Read the model definition and answer for the solid it produces. Units are mm, in the model's axes. Face numbers are marked on the shaded views. A direction names the side the tool comes from. Round coordinates to 2 decimals unless told otherwise and drop trailing zeros. Loops run counter-clockwise (first coordinate to the right, second up) from the corner with the lowest first, then second, coordinate; pieces in that order, holes last. Notation, with made-up numbers: (61, -18) - (105, -18) arc R22 ccw to (105, 15) - close; hole circle Ø11 at (29.5, -11). An arc over 180 degrees is marked (long way). Answer as CSV lines item,"result".
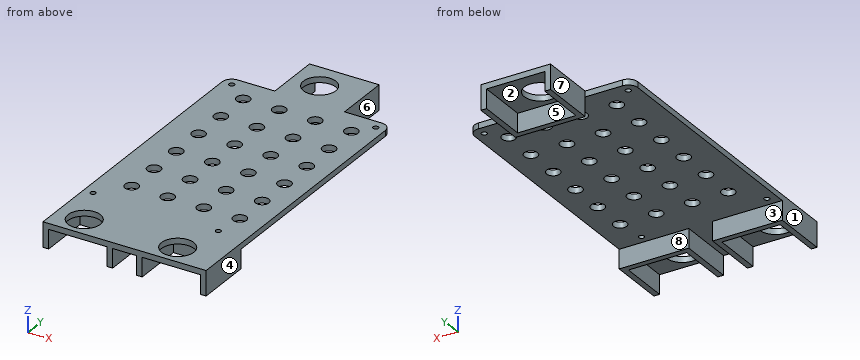
Autodesk Inventor part; units mm, degrees
ref_plane "Arbeitsebene2" through (-15.25, 66.75, 0) normal (0, 0, 1) x (1, 0, 0)
ref_plane "YZ Plane" through (0, 0, 0) normal (1, 0, 0) x (0, 1, 0)
ref_plane "XZ Plane" through (0, 0, 0) normal (0, 1, 0) x (-1, 0, 0)
ref_plane "Arbeitsebene1" through (0, 0, 0) normal (0, 0, 1) x (1, 0, 0)
sketch "Skizze1" plane through (0, 0, 0) normal (0, 0, 1) x (1, 0, 0)
  arc A0 (-36.75, 55.75) -> (-34.75, 57.75) centre (-36.75, 57.75) ccw
  line L0 (-34.75, 57.75) -> (-34.75, 60.25)
  arc A1 (-32.75, 62.25) -> (-34.75, 60.25) centre (-32.75, 60.25) ccw
  line L1 (-32.75, 62.25) -> (32.25, 62.25)
  arc A2 (34.25, 60.25) -> (32.25, 62.25) centre (32.25, 60.25) ccw
  line L2 (34.25, 60.25) -> (34.25, 57.25)
  arc A3 (34.25, 57.25) -> (36.25, 55.25) centre (36.25, 57.25) ccw
  line L3 (36.25, 55.25) -> (39.25, 55.25)
  arc A4 (41.25, 53.25) -> (39.25, 55.25) centre (39.25, 53.25) ccw
  line L4 (41.25, 53.25) -> (41.25, -58.75)
  arc A5 (37.75, -62.25) -> (41.25, -58.75) centre (37.75, -58.75) ccw
  line L5 (37.75, -62.25) -> (33.25, -62.25)
  arc A6 (31.25, -60.25) -> (33.25, -62.25) centre (33.25, -60.25) ccw
  line L6 (31.25, -60.25) -> (31.25, -57.25)
  arc A7 (31.25, -57.25) -> (29.25, -55.25) centre (29.25, -57.25) ccw
  line L7 (29.25, -55.25) -> (26.25, -55.25)
  arc A8 (26.25, -55.25) -> (24.25, -57.25) centre (26.25, -57.25) ccw
  line L8 (24.25, -57.25) -> (24.25, -60.25)
  arc A9 (22.25, -62.25) -> (24.25, -60.25) centre (22.25, -60.25) ccw
  line L9 (22.25, -62.25) -> (-30.5541, -62.25)
  arc A10 (-32.5541, -60.25) -> (-30.5541, -62.25) centre (-30.5541, -60.25) ccw
  line L10 (-32.5541, -60.25) -> (-32.5541, -56.8048)
  arc A11 (-32.5541, -56.8048) -> (-34.5541, -54.8048) centre (-34.5541, -56.8048) ccw
  line L11 (-34.5541, -54.8048) -> (-39.25, -54.8048)
  arc A12 (-41.25, -52.8048) -> (-39.25, -54.8048) centre (-39.25, -52.8048) ccw
  line L12 (-41.25, -52.8048) -> (-41.25, 53.75)
  arc A13 (-39.25, 55.75) -> (-41.25, 53.75) centre (-39.25, 53.75) ccw
  line L13 (-39.25, 55.75) -> (-36.75, 55.75)
  line L14 (42.75, -58.75) -> (42.75, 58.75)
  arc A14 (42.75, 58.75) -> (37.75, 63.75) centre (37.75, 58.75) ccw
  line L15 (37.75, 63.75) -> (-37.75, 63.75)
  arc A15 (-37.75, 63.75) -> (-42.75, 58.75) centre (-37.75, 58.75) ccw
  line L16 (-42.75, 58.75) -> (-42.75, -58.75)
  arc A16 (-42.75, -58.75) -> (-37.75, -63.75) centre (-37.75, -58.75) ccw
  line L17 (-37.75, -63.75) -> (37.75, -63.75)
  arc A17 (37.75, -63.75) -> (42.75, -58.75) centre (37.75, -58.75) ccw
  circle A18 centre (-37.75, 58.75) radius 1.4
  circle A19 centre (-37.75, -58.75) radius 1.4
  circle A20 centre (37.75, 58.75) radius 1.4
  circle A21 centre (28.25, -59.25) radius 1.4
  point P0 (0, 0)
extrude "Extrusion1" add sketch "Skizze1" along normal blind 3 contours A0 L0 A1 L1 A2 L2 A3 L3 A4 L4 A5 L5 A6 L6 A7 L7 A8 L8 A9 L9 A10 L10 A11 L11 A12 L12 A13 L13 | A17 L17 A16 L16 A15 L15 A14 L14
sketch "Skizze2" plane through (0, 0, 3) normal (0, 0, 1) x (1, 0, 0)
  circle A0 centre (-26.4114, 50.1197) radius 3.8655 construction
  circle A1 centre (-26.4114, 50.1197) radius 3.5
  point P0 (0, 0)
  dimension "d2" = 7
extrude "Extrusion2" cut sketch "Skizze2" against normal through all
pattern_linear "Rechteckige Anordnung1" count 6 spacing 18.9 along (0, -1, 0) count 4 spacing 18.9 along (1, 0, 0) of "Extrusion2"
sketch "Skizze3" plane through (0, 0, 3) normal (0, 0, 1) x (1, 0, 0)
  circle A0 centre (-28.25, -81.65) radius 8.5
  line L0 (-9.25, -66.75) -> (-39.75, -66.75)
  line L1 (-39.75, -66.75) -> (-39.75, -93.15)
  line L2 (-39.75, -93.15) -> (-9.25, -93.15)
  line L3 (-9.25, -93.15) -> (-9.25, -66.75)
  circle A1 centre (-3.75, 78.25) radius 8.5
  line L4 (15.25, 93.15) -> (-15.25, 93.15)
  line L5 (-15.25, 93.15) -> (-15.25, 66.75)
  line L6 (-15.25, 66.75) -> (15.25, 66.75)
  line L7 (15.25, 66.75) -> (15.25, 93.15)
  circle A2 centre (20.75, -81.65) radius 8.5
  line L8 (39.75, -66.75) -> (9.25, -66.75)
  line L9 (9.25, -66.75) -> (9.25, -93.15)
  line L10 (9.25, -93.15) -> (39.75, -93.15)
  line L11 (39.75, -93.15) -> (39.75, -66.75)
  line L12 (-42.75, 58.75) -> (-42.75, -58.75)
  line L13 (-42.75, -66.75) -> (-42.75, -58.75)
  line L14 (-42.75, -58.75) -> (-41.9493, -58.75)
  line L15 (-9.25, -93.15) -> (9.25, -93.15)
  arc A3 (37.75, -63.75) -> (42.75, -58.75) centre (37.75, -58.75) ccw
  line L16 (42.75, -66.75) -> (42.75, -58.75)
  line L17 (37.75, 63.75) -> (-37.75, 63.75)
  line L18 (-15.25, 93.15) -> (15.25, 93.15)
  line L19 (15.25, 93.15) -> (15.25, 63.75)
  line L20 (15.25, 63.75) -> (-15.25, 63.75)
  line L21 (-15.25, 63.75) -> (-15.25, 93.15)
  arc A4 (-42.75, -58.75) -> (-37.75, -63.75) centre (-37.75, -58.75) ccw
  circle A5 centre (30.2886, -44.3803) radius 3.5
  circle A6 centre (30.2886, -25.4803) radius 3.5
  circle A7 centre (30.2886, -6.5803) radius 3.5
  circle A8 centre (30.2886, 12.3197) radius 3.5
  circle A9 centre (30.2886, 31.2197) radius 3.5
  circle A10 centre (30.2886, 50.1197) radius 3.5
  circle A11 centre (11.3886, -44.3803) radius 3.5
  circle A12 centre (11.3886, -25.4803) radius 3.5
  circle A13 centre (11.3886, -6.5803) radius 3.5
  circle A14 centre (11.3886, 12.3197) radius 3.5
  circle A15 centre (11.3886, 31.2197) radius 3.5
  circle A16 centre (11.3886, 50.1197) radius 3.5
  circle A17 centre (-7.5114, -44.3803) radius 3.5
  circle A18 centre (-7.5114, -25.4803) radius 3.5
  circle A19 centre (-7.5114, -6.5803) radius 3.5
  circle A20 centre (-7.5114, 12.3197) radius 3.5
  circle A21 centre (-7.5114, 31.2197) radius 3.5
  circle A22 centre (-7.5114, 50.1197) radius 3.5
  circle A23 centre (-26.4114, -44.3803) radius 3.5
  circle A24 centre (-26.4114, -25.4803) radius 3.5
  circle A25 centre (-26.4114, -6.5803) radius 3.5
  circle A26 centre (-26.4114, 12.3197) radius 3.5
  circle A27 centre (-26.4114, 31.2197) radius 3.5
  circle A28 centre (-26.4114, 50.1197) radius 3.5
  arc A29 (42.75, 58.75) -> (37.75, 63.75) centre (37.75, 58.75) ccw
  line L22 (37.75, 63.75) -> (-37.75, 63.75)
  arc A30 (-37.75, 63.75) -> (-42.75, 58.75) centre (-37.75, 58.75) ccw
  line L23 (-42.75, 58.75) -> (-42.75, -58.75)
  arc A31 (-42.75, -58.75) -> (-37.75, -63.75) centre (-37.75, -58.75) ccw
  line L24 (-37.75, -63.75) -> (37.75, -63.75)
  arc A32 (37.75, -63.75) -> (42.75, -58.75) centre (37.75, -58.75) ccw
  line L25 (42.75, -58.75) -> (42.75, 58.75)
  circle A33 centre (28.25, -59.25) radius 1.4
  circle A34 centre (37.75, 58.75) radius 1.4
  circle A35 centre (-37.75, -58.75) radius 1.4
  circle A36 centre (-37.75, 58.75) radius 1.4
  line L26 (15.25, 93.15) -> (18.25, 93.15)
  line L27 (18.25, 93.15) -> (18.25, 63.75)
  line L28 (18.25, 63.75) -> (15.25, 63.75)
  line L29 (15.25, 63.75) -> (15.25, 93.15)
  line L30 (-15.25, 93.15) -> (-18.25, 93.15)
  line L31 (-18.25, 93.15) -> (-18.25, 63.75)
  line L32 (-18.25, 63.75) -> (-15.25, 63.75)
  line L33 (-15.25, 63.75) -> (-15.25, 93.15)
  line L34 (-39.75, -93.15) -> (-42.75, -93.15)
  line L35 (-42.75, -93.15) -> (-42.75, -58.75)
  line L36 (-42.75, -58.75) -> (-39.75, -58.75)
  line L37 (-39.75, -58.75) -> (-39.75, -93.15)
  line L38 (39.75, -93.15) -> (42.75, -93.15)
  line L39 (42.75, -93.15) -> (42.75, -58.75)
  line L40 (42.75, -58.75) -> (39.75, -58.75)
  line L41 (39.75, -58.75) -> (39.75, -93.15)
  point P0 (0, 0)
  point P1 (15.25, 66.75)
  point P2 (-15.25, 63.75)
  point P3 (41.5171, -62.0377)
  point P4 (42.75, -58.75)
  point P5 (42.75, -58.75)
  point P6 (-41.5171, -62.0377)
  point P7 (42.75, -58.75)
  point P8 (41.5171, -62.0377)
  point P9 (42.75, -58.75)
  point P10 (-37.75, 63.75)
  dimension "d17" = 3
  dimension "d18" = 3
ref_plane "Arbeitsebene2" through (-15.25, 66.75, 0) normal (0, 0, 1) x (1, 0, 0)
extrude "Extrusion3" add sketch "Skizze3" against normal up to surface (3 mm away)
sketch "Skizze4" plane through (0, 0, 0) normal (0, 0, -1) x (-1, 0, 0)
  circle A0 centre (19.25, -88.65) radius 0.65
  line L0 (9.25, -93.15) -> (9.25, -66.75)
  line L1 (9.25, -66.75) -> (39.75, -66.75)
  line L2 (-9.25, -66.75) -> (-9.25, -93.15)
  line L3 (-39.75, -66.75) -> (-9.25, -66.75)
  line L4 (15.25, 66.75) -> (-15.25, 66.75)
  line L5 (-37.75, 63.75) -> (37.75, 63.75)
  line L6 (-15.25, 66.75) -> (15.25, 66.75)
  line L7 (15.25, 66.75) -> (15.25, 63.75)
  line L8 (15.25, 63.75) -> (-15.25, 63.75)
  line L9 (-15.25, 63.75) -> (-15.25, 66.75)
  line L10 (9.25, -93.15) -> (6.25, -93.15)
  line L11 (6.25, -93.15) -> (6.25, -63.7252)
  line L12 (6.25, -63.7252) -> (9.25, -63.7252)
  line L13 (9.25, -63.7252) -> (9.25, -93.15)
  line L14 (-9.25, -93.15) -> (-6.25, -93.15)
  line L15 (-6.25, -93.15) -> (-6.25, -63.7252)
  line L16 (-6.25, -63.7252) -> (-9.25, -63.7252)
  line L17 (-9.25, -63.7252) -> (-9.25, -93.15)
  line L18 (42.75, 58.75) -> (42.75, -93.15)
  line L19 (-42.75, 58.75) -> (-42.75, -93.15)
  line L20 (-9.25, -66.75) -> (-39.75, -66.75)
  line L21 (-39.75, -66.75) -> (-39.75, -63.7252)
  line L22 (-39.75, -63.7252) -> (-9.25, -63.7252)
  line L23 (-9.25, -63.7252) -> (-9.25, -66.75)
  line L24 (42.75, 58.75) -> (42.75, -93.15)
  line L25 (9.25, -66.75) -> (42.75, -66.75)
  line L26 (42.75, -66.75) -> (42.75, -63.7252)
  line L27 (42.75, -63.7252) -> (9.25, -63.7252)
  line L28 (9.25, -63.7252) -> (9.25, -66.75)
  line L29 (-18.25, 93.15) -> (-18.25, 63.75)
  line L30 (18.25, 63.75) -> (18.25, 93.15)
  line L31 (-18.25, 93.15) -> (-15.25, 93.15)
  line L32 (-15.25, 93.15) -> (-15.25, 63.75)
  line L33 (-15.25, 63.75) -> (-18.25, 63.75)
  line L34 (-18.25, 63.75) -> (-18.25, 93.15)
  line L35 (18.25, 63.75) -> (37.75, 63.75)
  line L36 (18.25, 63.75) -> (15.25, 63.75)
  line L37 (15.25, 63.75) -> (15.25, 93.15)
  line L38 (15.25, 93.15) -> (18.25, 93.15)
  line L39 (18.25, 93.15) -> (18.25, 63.75)
  line L40 (-42.75, -93.15) -> (-42.75, 58.75)
  line L41 (-42.75, -93.15) -> (-39.75, -93.15)
  line L42 (-39.75, -93.15) -> (-39.75, -63.7252)
  line L43 (-39.75, -63.7252) -> (-42.75, -63.7252)
  line L44 (-42.75, -63.7252) -> (-42.75, -93.15)
  line L45 (42.75, -93.15) -> (39.75, -93.15)
  line L46 (39.75, -93.15) -> (39.75, -66.75)
  line L47 (39.75, -66.75) -> (42.75, -66.75)
  line L48 (42.75, -66.75) -> (42.75, -93.15)
  point P0 (0, 0)
  point P1 (9.25, -63.7252)
  point P2 (9.25, -66.75)
  point P3 (-9.25, -63.7252)
  point P4 (-42.75, -63.7252)
  point P5 (-9.25, -66.75)
  point P6 (-9.25, -63.7252)
  point P7 (-42.75, -58.75)
  point P8 (42.75, -58.75)
  dimension "d13" = 3
  dimension "d14" = 3
extrude "Extrusion4" add sketch "Skizze4" along normal blind 10 contours L10 L11 L12 L13 L0 | L13 L27 L18 L25 L1 | L25 L18 L45 L46 | L17 L16 L15 L14 L2 | L3 L21 L22 L17 | L42 L41 L19 L43 L21 | L7 L5 L9 L4 | L37 L38 L30 L5 L7 | L9 L5 L29 L31 L32
properties part number "Omniscope_lensmount_v0"
1) The mould has two halves that part along X. Classify the marked faces 1, 2, 3 and 4: pulls with the +X half, pulls with the -X half, needs draft (parallel to the pull), parting line crosses it, or undercut.
Entries:
face 1,"pulls with the -X half"
face 2,"undercut"
face 3,"needs draft"
face 4,"pulls with the +X half"
2) Find the intervals of material crossed by line 1 (X direction, y = 81.5, z = -7.75); line 2 (Y direction, x = 37.75, z = 2.1); line 3 (Y direction, x = -37.75, z = 1.4), in increasing order.
Entries:
line 1,"x = -18.25 to -15.25, 15.25 to 18.25"
line 2,"y = -93.15 to 57.35, 60.15 to 63.75"
line 3,"y = -93.15 to -60.15, -57.35 to 57.35, 60.15 to 63.75"
3) A cutting plane is placed at B-B, the plane y = -81.65. Determine the outline of the cut face in (x, z), plus the area to 4 significant figures.
Entries:
outline,"(-42.75, -10) - (-39.75, -10) - (-39.75, 0) - (-36.75, 0) - (-36.75, 3) - (-42.75, 3) - close; (-19.75, 0) - (-9.25, 0) - (-9.25, -10) - (-6.25, -10) - (-6.25, 0) - (6.25, 0) - (6.25, -10) - (9.25, -10) - (9.25, 0) - (12.25, 0) - (12.25, 3) - (-19.75, 3) - close; (29.25, 0) - (39.75, 0) - (39.75, -10) - (42.75, -10) - (42.75, 3) - (29.25, 3) - close"
area,"274.5 mm^2"
4) A cutting plane is placed at A-A, the plane z = -5. Determine the outline of the cut face in (x, y).
Entries:
outline,"(-42.75, -93.15) - (-39.75, -93.15) - (-39.75, -66.75) - (-9.25, -66.75) - (-9.25, -93.15) - (-6.25, -93.15) - (-6.25, -63.73) - (-42.75, -63.73) - close; (-18.25, 63.75) - (18.25, 63.75) - (18.25, 93.15) - (15.25, 93.15) - (15.25, 66.75) - (-15.25, 66.75) - (-15.25, 93.15) - (-18.25, 93.15) - close; (6.25, -93.15) - (9.25, -93.15) - (9.25, -66.75) - (39.75, -66.75) - (39.75, -93.15) - (42.75, -93.15) - (42.75, -63.73) - (6.25, -63.73) - close"
5) Each of these flat-tipped pins is pushed along its axis until it touches: P1, Ø4, axis at x = -7.51, y = 50.12, coming from the +Z side; P2, Ø5, axis at x = 21.5, z = -7, coming from the -Y side; P3, Ø13, axis at x = 31.5, y = -84, coming from the -Z side. Where does it stop, or does it pass through?
Entries:
P1,"passes through"
P2,"stops at y = -66.75"
P3,"stops at z = 0"
6) A tool of negligible diameter and unlimited length cuts with its end or side. For the marked faces 5, 6, 7 and 8, from which of +Z, -Z, +X, -X, +Y, -Y can it reach the whole face along a straight path? Write none if from no direction.
Entries:
face 5,"-Z, +Y"
face 6,"+Z, -Z, +X, +Y"
face 7,"+Z, -Z, -X, +Y"
face 8,"-Z, +X, -X"
7) A cutting plane is placed at C-C, the plane x = 20.5. Determine the outline of the cut face in (y, z).
Entries:
outline,"(-93.15, 0) - (-90.15, 0) - (-90.15, 3) - (-93.15, 3) - close; (-73.15, 0) - (-66.75, 0) - (-66.75, -10) - (-63.73, -10) - (-63.73, 0) - (63.75, 0) - (63.75, 3) - (-73.15, 3) - close"
